Autodesk Inventor part; units mm, degrees
ref_plane "YZ Plane" through (0, 0, 0) normal (1, 0, 0) x (0, 1, 0)
ref_plane "XZ Plane" through (0, 0, 0) normal (0, 1, 0) x (-1, 0, 0)
ref_plane "XY Plane" through (0, 0, 0) normal (0, 0, 1) x (1, 0, 0)
sketch "Sketch1" plane through (0, 0, 0) normal (0, 0, 1) x (1, 0, 0)
  line L0 (-18.3251, 8.6116) -> (32.4749, 8.6116)
  line L1 (32.4749, 8.6116) -> (32.4749, -29.4884)
  line L2 (32.4749, -29.4884) -> (-18.3251, -29.4884)
  line L3 (-18.3251, -29.4884) -> (-18.3251, 8.6116)
  point P0 (0, 0)
  dimension "d0" = 50.8
  dimension "d1" = 38.1
extrude "Extrusion1" add sketch "Sketch1" along normal blind 31.75
sketch "Sketch2" plane through (-18.3251, 8.6116, 0) normal (0, 1, 0) x (1, 0, 0)
  line L0 (50.8, -31.75) -> (0, -31.75)
  line L1 (12.7, -31.75) -> (38.1, -31.75)
  line L2 (38.1, -31.75) -> (38.1, -19.05)
  line L3 (38.1, -19.05) -> (12.7, -19.05)
  line L4 (12.7, -19.05) -> (12.7, -31.75)
  line L5 (50.8, 0) -> (50.8, -31.75)
  point P0 (18.3251, 0)
  dimension "d4" = 12.7
  dimension "d5" = 25.4
  dimension "d6" = 12.7
extrude "Extrusion2" cut sketch "Sketch2" against normal blind 38.1
sketch "Sketch3" plane through (0, 0, 31.75) normal (0, 0, 1) x (1, 0, 0)
  line L0 (32.4749, -29.4884) -> (32.4749, 8.6116)
  line L1 (19.7749, 8.6116) -> (32.4749, 8.6116)
  line L2 (32.4749, 8.6116) -> (32.4749, -10.4384)
  line L3 (32.4749, -10.4384) -> (19.7749, -10.4384)
  line L4 (19.7749, -10.4384) -> (19.7749, 8.6116)
  line L5 (-5.6251, 8.6116) -> (-18.3251, 8.6116)
  line L6 (-5.6251, -29.4884) -> (-5.6251, 8.6116)
  line L7 (-18.3251, 8.6116) -> (-5.6251, 8.6116)
  line L8 (-5.6251, 8.6116) -> (-5.6251, -10.4384)
  line L9 (-5.6251, -10.4384) -> (-18.3251, -10.4384)
  line L10 (-18.3251, -10.4384) -> (-18.3251, 8.6116)
  line L11 (-18.3251, -29.4884) -> (-5.6251, -29.4884)
  line L12 (19.7749, -29.4884) -> (32.4749, -29.4884)
  point P0 (0, 0)
  dimension "d9" = 19.05
  dimension "d10" = 19.05
extrude "Extrusion3" cut sketch "Sketch3" against normal blind 38.1
properties part number "Figure 7_27_7"
The listing builds one solid part. Answer for the finished solid, in the listing's coordinates (mm). A direction names the side the tool comes from. Give positions to 0.01 mm unless a question says otherwise; leave off trailing zeros. Order: outer loops, then holes, each group sorted by start corner. A loop starts at its lowest first (then second) coordinate and runs counter-clockwise, first axis right, second up. Notation, with made-up numbers: (-19, 16) -> (21, 16) arc R15 cw to (21, 38) -> close; hole circle Ø9 at (87.5, 53.25). An arc over 180 degrees is marked (long way). One line per item, written item: value.
1) Flat-ended cylindrical pins translate along their axes: P1, Ø6.5, axis at x = 28, z = 22.5, coming from the +Y side; P2, Ø1, axis at x = -7, y = -3.5, coming from the -Z side; P3, Ø15, axis at y = 3, z = 9, coming from the +X side; P4, Ø5.5, axis at y = 1, z = 14, coming from the -X side. Find the tip coordinate at first contact, or state that the pin passes through.
Reported:
P1: stops at y = -10.44
P2: passes through
P3: stops at x = 19.77
P4: stops at x = -5.63
2) A tool of negligible diameter and unlimited length cuts with its end or side. For faces 1 (the flat face through (-5.625, -20, 25)), 2 (the flat face through (-12, -10.438, 16)), 3 (the flat face through (7, -29.488, 12)), 4 (the flat face through (19.775, -1, 10)), from which of +Z, -Z, +X, -X, +Y, -Y can it reach the whole face along a straight path? Write none if from no direction.
Reported:
face 1: +Z, +Y, -Y
face 2: +Z, -Z, -X, +Y
face 3: +Z, -Z, +X, -X, -Y
face 4: +Z, -Z, +X, +Y
3) Find section B-B, the plane y = -23. Determine the outline of the cut face in (x, z).
Reported:
outline: (-18.33, 0) -> (32.47, 0) -> (32.47, 31.75) -> (19.77, 31.75) -> (19.77, 19.05) -> (-5.63, 19.05) -> (-5.63, 31.75) -> (-18.33, 31.75) -> close
4) Find section D-D, the plane x = -12.5. Determine the outline of the cut face in (y, z), plus the area to 3 significant figures.
Reported:
outline: (-29.49, 0) -> (-10.44, 0) -> (-10.44, 31.75) -> (-29.49, 31.75) -> close
area: 605 mm^2
5) Find the intervals of material crossed by line 1 (X direction, y = -15, z = 22); line 2 (Y direction, x = -8.5, z = 11); line 3 (Z direction, x = -5, y = -13), in increasing order.
Reported:
line 1: x = -18.33 to -5.63, 19.77 to 32.47
line 2: y = -29.49 to -10.44
line 3: z = 0 to 19.05
6) Find section A-A, the plane z = 21.5. Determine the outline of the cut face in (x, y).
Reported:
outline: (-18.33, -29.49) -> (-5.63, -29.49) -> (-5.63, -10.44) -> (-18.33, -10.44) -> close; (19.77, -29.49) -> (32.47, -29.49) -> (32.47, -10.44) -> (19.77, -10.44) -> close
7) Find section C-C, the plane z = 14. Determine the outline of the cut face in (x, y).
Reported:
outline: (-18.33, -29.49) -> (32.47, -29.49) -> (32.47, -10.44) -> (19.77, -10.44) -> (19.77, 8.61) -> (-5.63, 8.61) -> (-5.63, -10.44) -> (-18.33, -10.44) -> close
8) Determine the mould class of faces 5 (the flat face through (-5.625, -1, 10)), 6 (the flat face through (19.775, -20, 25)), 7 (the flat face through (7, -10, 19.05)), 8 (the flat face through (7, 8.612, 9)) for opening direction X: pulls with the +X half, pulls with the -X half, needs draft (parallel to the pull), parting line crosses it, or undercut.
Reported:
face 5: pulls with the -X half
face 6: undercut
face 7: undercut
face 8: needs draft
